```python
from build123d import *

# Parameters (mm, degrees)
F0_W     = 949.2
F0_H     = 50.8
F0_W_2   = 50.8
F0_H_2   = 949.2
F1_DEPTH = 1000
F3_DEPTH = 1800
F5_DEPTH = 5360
F7_START = 131
F7_DEPTH = 629


with BuildPart() as f1:
    # F0 (on Right) → F1 (new body)
    with BuildSketch(Plane.YZ):
        with Locations((-29.1286933511, 973.496588254)):
            Rectangle(F0_W, F0_H)
        with Locations((470.8713066489, 973.496588254)):
            Rectangle(F0_W_2, F0_H)
        with Locations((470.8713066489, 1473.496588254)):
            Rectangle(F0_W_2, F0_H_2)
        Polygon((-503.7286933511, -1.103411746), (-503.7286933511, -51.903411746), (496.2713066489, -51.903411746), (496.2713066489, 948.096588254), (445.4713066489, 948.096588254), (445.4713066489, 0), align=None)
    extrude(amount=F1_DEPTH)

    # F2 (on Top) → F3 (join)
    with BuildSketch(Plane.XY):
        with BuildLine():
            ThreePointArc((857.5784564018, -130.1132158098), (896.2008242629, -181.7113174116), (913.260281086, -243.8645660877))
            Line((913.260281086, -243.8645660877), (913.260281086, 360.6808781624))
            Line((913.260281086, 360.6808781624), (857.5784564018, 360.6808781624))
            Line((857.5784564018, 360.6808781624), (857.5784564018, -130.1132158098))
        make_face()
        with BuildLine():
            ThreePointArc((611.3790712788, -372.640659557), (668.6957081838, -415.0795417944), (738.2603287697, -430.7963848114))
            ThreePointArc((738.2603287697, -430.7963848114), (862.2437509886, -381.0271980017), (913.8211489182, -257.785025984))
            ThreePointArc((913.8211489182, -257.785025984), (913.6808751008, -250.8191488596), (913.260281086, -243.8645660877))
            ThreePointArc((913.260281086, -243.8645660877), (896.2008242629, -181.7113174116), (857.5784564018, -130.1132158098))
            Line((857.5784564018, -130.1132158098), (857.5784564018, -243.8645660877))
            ThreePointArc((857.5784564018, -243.8645660877), (858.1982990198, -250.8125329656), (858.4051557693, -257.785025984))
            ThreePointArc((858.4051557693, -257.785025984), (823.0571563331, -341.8406590918), (738.2603287697, -375.3716679713))
            Line((738.2603287697, -375.3716679713), (611.3790712788, -372.640659557))
        make_face()
        with BuildLine():
            Line((292.8057610989, -365.7836468832), (292.8057610989, -430.7963848114))
            Line((292.8057610989, -430.7963848114), (738.2603287697, -430.7963848114))
            ThreePointArc((738.2603287697, -430.7963848114), (668.6957081838, -415.0795417944), (611.3790712788, -372.640659557))
            Line((611.3790712788, -372.640659557), (292.8057610989, -365.7836468832))
        make_face()
    extrude(amount=F3_DEPTH)

    # F4 (on Right) → F5 (cut)
    with BuildSketch(Plane.YZ):
        with BuildLine():
            Line((-435.6626272202, 1808.1647157669), (-436.3610964974, 1002.8872649632))
            Line((-436.3610964974, 1002.8872649632), (96.866071558, 1002.8872649632))
            Line((96.866071558, 1002.8872649632), (202.9513269663, 1646.3969945908))
            add(Edge.make_bspline(
                [(202.9513269663, 1646.3969945908), (204.5801297554, 1657.9332047918), (208.2046485199, 1683.6043361435), (225.3759496446, 1736.6871062603), (256.9211367372, 1774.2470270708), (280.5041077395, 1798.206239093), (317.8181539373, 1801.9341732886), (350.8337600962, 1795.8752573669), (357.6071157247, 1788.8956994391), (360.1746559143, 1786.2499952316)],
                knots=[0, 0, 0, 0, 0.1468911817, 0.3268718889, 0.4960081367, 0.6320686272, 0.7781002106, 0.9158856173, 1, 1, 1, 1], degree=3))
            Line((360.1746559143, 1786.2499952316), (360.1746559143, 1808.1647157669))
            Line((360.1746559143, 1808.1647157669), (-435.6626272202, 1808.1647157669))
        make_face()
        with BuildLine():
            Line((-436.4086301738, 948.084857743), (-436.8441998959, 445.9089040756))
            Line((-436.8441998959, 445.9089040756), (-348.0192422867, 445.9089040756))
            Line((-348.0192422867, 445.9089040756), (-243.5122281313, 445.9089040756))
            Line((-243.5122281313, 445.9089040756), (-243.5122281313, 220.3548997641))
            add(Edge.make_bspline(
                [(-243.5122281313, 220.3548997641), (-233.785627989, 201.848121656), (-224.0590278467, 183.3413435479), (-211.8256313009, 166.9237262564)],
                knots=[0, 0, 0, 0, 0.1915955458, 0.1915955458, 0.1915955458, 0.1915955458], degree=3))
            Line((-211.8256313009, 166.9237262564), (-179.0682524443, 134.4295740128))
            Line((-179.0682524443, 134.4295740128), (-64.2616951351, 134.4295740128))
            add(Edge.make_bspline(
                [(-64.2616951351, 134.4295740128), (-48.6215669755, 155.0982523243), (-40.3796052607, 187.7265760442), (-32.1376435459, 220.3548997641)],
                knots=[0.7406470598, 0.7406470598, 0.7406470598, 0.7406470598, 1, 1, 1, 1], degree=3))
            Line((-32.1376435459, 220.3548997641), (87.7567170793, 947.630215196))
            Line((87.7567170793, 947.630215196), (-436.4086301738, 948.084857743))
        make_face()
        with BuildLine():
            Line((-243.5122281313, 445.9089040756), (-348.0192422867, 445.9089040756))
            Line((-348.0192422867, 445.9089040756), (-348.0192422867, 302.02293396))
            Line((-348.0192422867, 302.02293396), (-211.8256313009, 166.9237262564))
            add(Edge.make_bspline(
                [(-243.5122281313, 220.3548997641), (-233.785627989, 201.848121656), (-224.0590278467, 183.3413435479), (-211.8256313009, 166.9237262564)],
                knots=[0, 0, 0, 0, 0.1915955458, 0.1915955458, 0.1915955458, 0.1915955458], degree=3))
            Line((-243.5122281313, 220.3548997641), (-243.5122281313, 445.9089040756))
        make_face()
    extrude(amount=F5_DEPTH, mode=Mode.SUBTRACT)

    # F6 (on Front) → F7 (cut)
    with BuildSketch(Plane.XZ.offset(F7_START)):
        Polygon((293.0140197277, 459.7436785698), (293.0140197277, 445.7174837589), (737.5785708427, 347.7625846863), (912.6507639885, 219.5038050413), (912.6507639885, 459.7436785698), align=None)
    extrude(amount=F7_DEPTH, mode=Mode.SUBTRACT)


solid = f1.part
```
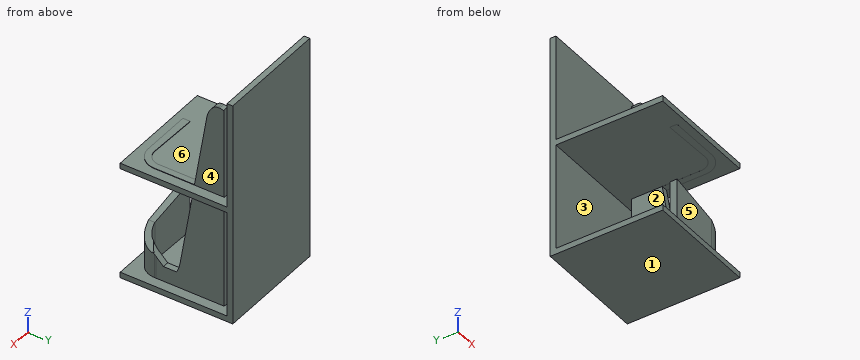
Geometry: final body of the model. Coordinates: model frame, mm. Face numbers are marked on the shaded views. A direction names the side the tool comes from. Round coordinates to 2 decimals unless told otherwise and drop trailing zeros. Loops run counter-clockwise (first coordinate to the right, second up) from the corner with the lowest first, then second, coordinate; pieces in that order, holes last. Notation, with made-up numbers: (-5, 70) -> (5, 70) arc R29 cw to (5, 101) -> close; hole circle Ø8 at (25.5, 7). An arc over 180 degrees is marked (long way). Write each question's results on one line, items separated by ' | '.
Item 1: Set-up query: the marked faces 1, 2 and 3. Return all of +Z, -Z, +X, -X, +Y, -Y with unobstructed straight access to the full face (end or side cutting, diameter ignored); none if empty.
Answers below:
face 1: -Z, +X, -X, +Y, -Y | face 2: -X | face 3: +X, -X
Item 2: Cut plane C-C on z = 391. Return the cut outline in (x, y).
Answers below:
outline: (0, 445.47) -> (1000, 445.47) -> (1000, 496.27) -> (0, 496.27) -> close; (292.81, -430.8) -> (541.35, -430.8) -> (541.35, -371.13) -> (292.81, -365.78) -> close; (857.58, -4.01) -> (913.26, -4.01) -> (913.26, 360.68) -> (857.58, 360.68) -> close
Item 3: Cut plane D-D on z = 713.5. Return the cut outline in (x, y), and give its area (3 significant figures).
Answers below:
outline: (0, 445.47) -> (1000, 445.47) -> (1000, 496.27) -> (0, 496.27) -> close; (857.58, 49.16) -> (913.26, 49.16) -> (913.26, 360.68) -> (857.58, 360.68) -> close | area: 68,100 mm²
Item 4: Cut plane B-B on y = 395. Return the cut outline in (x, z), and give its area (3 significant figures).
Answers below:
outline: (0, -51.9) -> (1000, -51.9) -> (1000, -0.06) -> (0, -0.06) -> close; (0, 948.1) -> (1000, 948.1) -> (1000, 998.9) -> (0, 998.9) -> close | area: 103,000 mm²
Item 5: Line query: probe 1 along Z at (x, y) = (221, -120); probe 2 along Z at (x, y) = (145, 289); probe 3 along Y at (x, z) = (52, 743). Output: solid intervals per line, ascending. Write a range as [from, to].
Answers below:
probe 1: z = [-51.9, -0.66], [948.1, 998.9] | probe 2: z = [-51.9, -0.18], [948.1, 998.9] | probe 3: y = [445.47, 496.27]
Item 6: Pin query (flat end, axial travel): pin 1 Ø1.5 at (x, z) = (699.5, 356) entering from -Y; pin 2 Ø1 at (y, z) = (200.5, 1443) entering from +X; pin 3 Ø1.2 at (y, z) = (-389, 1001) entering from -X; pin 4 Ø4.5 at (x, z) = (428.5, 1000.5) entering from -Y. Return the tip coordinate at first contact, or that it passes through.
Answers below:
pin 1: stops at y = -430.8 | pin 2: stops at x = 913.26 | pin 3: stops at x = 292.81 | pin 4: stops at y = -503.73
Item 7: Pull-direction query (Y, two-part tool) for the marked faces 4, 5 and 6; classes: pulls with the +Y half, pulls with the -Y half, needs draft (parallel to the pull), parting line crosses it, or undercut.
Answers below:
face 4: needs draft | face 5: pulls with the -Y half | face 6: undercut
